Input: part model. Units: mm. Frame: model coordinates. Face numbers are marked on the shaded views. A direction names the side the tool comes from. Round coordinates to 2 decimals unless told otherwise and drop trailing zeros. Order: outer loops, then holes, each group sorted by start corner. A loop starts at its lowest first (then second) coordinate and runs counter-clockwise, first axis right, second up. Notation, with made-up numbers: (78, 61) -> (130, 61) arc R28 cw to (130, 87) -> close; hole circle Ø7 at (-32.5, 72.25). An arc over 180 degrees is marked (long way). Use a Markdown table: item, result.
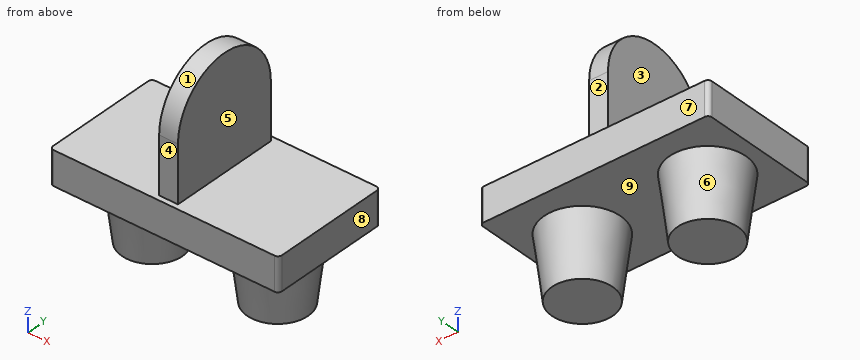
Autodesk Inventor part; units mm, degrees
ref_plane "YZ Plane" through (0, 0, 0) normal (1, 0, 0) x (0, 1, 0)
ref_plane "XZ Plane" through (0, 0, 0) normal (0, 1, 0) x (-1, 0, 0)
ref_plane "XY Plane" through (0, 0, 0) normal (0, 0, 1) x (1, 0, 0)
sketch "Sketch1" plane through (0, 0, 0) normal (0, 0, 1) x (1, 0, 0)
  line L0 (-7.3, 3.875) -> (7.3, 3.875)
  line L1 (7.3, 3.875) -> (7.3, -3.875)
  line L2 (7.3, -3.875) -> (-7.3, -3.875)
  line L3 (-7.3, -3.875) -> (-7.3, 3.875)
  point P0 (0, 0)
  point P1 (-7.3, 0)
  point P2 (0, 3.875)
  dimension "d0" = 14.6
  dimension "d1" = 7.75
extrude "Extrusion1" add sketch "Sketch1" along normal mid plane 2.15
fillet "Fillet1" radius 0.25 4 edges at (-7.3, 3.875, 0) (-7.3, -3.875, 0) (7.3, 3.875, 0) (7.3, -3.875, 0)
sketch "Sketch2" plane through (0, 0, 0) normal (1, 0, 0) x (0, 1, 0)
  line L0 (3.625, 1.075) -> (-3.625, 1.075) construction
  line L1 (3.54, 1.075) -> (3.54, 4.675)
  arc A0 (3.54, 4.675) -> (-3.54, 4.675) centre (0, 4.675) ccw
  line L2 (-3.54, 4.675) -> (-3.54, 1.075)
  line L3 (-3.54, 1.075) -> (3.54, 1.075)
  point P0 (0, 0)
  dimension "d5" = 3.6
  dimension "d6" = 7.08
extrude "Extrusion2" add sketch "Sketch2" along normal mid plane 1.2
sketch "Sketch3" plane through (0, 0, 0) normal (0, 1, 0) x (-1, 0, 0)
  line L0 (7.05, -1.075) -> (-7.05, -1.075) construction
  line L1 (-4, -1.075) -> (-6.44, -1.075)
  line L2 (-6.44, -1.075) -> (-5.94, -5.075)
  line L3 (-5.94, -5.075) -> (-4, -5.075)
  line L4 (-4, -5.075) -> (-4, -1.075)
  point P0 (0, 0)
  dimension "d9" = 4.88
  dimension "d10" = 3.88
  dimension "d11" = 4
  dimension "d12" = 4
revolve "Revolution1" add sketch "Sketch3" angle 360 about axis through (4, 0, -5.075) along (0, 0, 1)
mirror "Mirror1" about plane through (0, 0, 0) normal (1, 0, 0) of "Revolution1"
properties part number "HIPS" material "250"
1) Line query: L1, parallel to Z at x = -5.5, y = 3.5 (3 decimals); L2, parallel to Z at x = -3.25, y = -1 (3 decimals); L3, parallel to X at y = 2.25, z = 5.75. Output: solid intervals per line, ascending. Write a range as [from, to].
Results found:
| item | result |
|---|---|
| L1 | z = [-1.075, 1.075] |
| L2 | z = [-5.075, 1.075] |
| L3 | x = [-0.6, 0.6] |
2) Cut plane D-D on z = 4.5. Return loops of the section in (x, y), and give its area (3 significant figures).
Results found:
| item | result |
|---|---|
| outline | (-0.6, -3.54) -> (0.6, -3.54) -> (0.6, 3.54) -> (-0.6, 3.54) -> close |
| area | 8.50 mm² |
3) Pull-direction query (X, two-part tool) for the marked faces 6, 7, 8 and 9; classes: +X half, -X half, draft (parallel to the pull), parting line (faces both ways), or undercut.
Results found:
| item | result |
|---|---|
| face 6 | undercut |
| face 7 | draft |
| face 8 | +X half |
| face 9 | undercut |
4) Set-up query: the marked faces 1, 2, 3, 4 and 5. Return all of +Z, -Z, +X, -X, +Y, -Y with unobstructed straight access to the full face (end or side cutting, diameter ignored); none if empty.
Results found:
| item | result |
|---|---|
| face 1 | +Z, +X, -X |
| face 2 | +Z, +X, -X, +Y |
| face 3 | +Z, -X, +Y, -Y |
| face 4 | +Z, +X, -X, -Y |
| face 5 | +Z, +X, +Y, -Y |
5) Cut plane B-B on x = 4. Return loops of the section in (y, z) (3 decimals), and give its area (3 significant figures).
Results found:
| item | result |
|---|---|
| outline | (-3.875, -1.075) -> (-2.44, -1.075) -> (-1.94, -5.075) -> (1.94, -5.075) -> (2.44, -1.075) -> (3.875, -1.075) -> (3.875, 1.075) -> (-3.875, 1.075) -> close |
| area | 34.2 mm² |
6) Pin query (flat end, axial travel): pin 1 Ø2 at (y, z) = (1.5, 4) entering from -X; pin 2 Ø2 at (y, z) = (0.5, 6) entering from +X; pin 3 Ø2.5 at (x, y) = (3.5, -2) entering from +Z (3 decimals). Return the tip coordinate at first contact, or that it passes through.
Results found:
| item | result |
|---|---|
| pin 1 | stops at x = -0.6 |
| pin 2 | stops at x = 0.6 |
| pin 3 | stops at z = 1.075 |
7) Cut plane C-C on z = -3. Return loops of the section in (x, y).
Results found:
| item | result |
|---|---|
| outline | circle Ø4.4 at (-4, 0); circle Ø4.4 at (4, 0) |
8) Cut plane A-A on y = 0. Return loops of the section in (x, z) (3 decimals).
Results found:
| item | result |
|---|---|
| outline | (-7.3, -1.075) -> (-6.44, -1.075) -> (-5.94, -5.075) -> (-2.06, -5.075) -> (-1.56, -1.075) -> (1.56, -1.075) -> (2.06, -5.075) -> (5.94, -5.075) -> (6.44, -1.075) -> (7.3, -1.075) -> (7.3, 1.075) -> (0.6, 1.075) -> (0.6, 8.215) -> (-0.6, 8.215) -> (-0.6, 1.075) -> (-7.3, 1.075) -> close |
